Geometry: final body of the model. Coordinates: model frame, mm. A direction names the side the tool comes from. Coordinates: 2 decimals unless noted, no trailing zeros. Write each loop counter-clockwise with the first axis right and the second up, starting at its lowest first coordinate (ties: lowest second). Pieces come first, ordered by that corner, then holes.
from build123d import *

# Parameters (mm, degrees)
CHAMFER_1_SIZE = 1


with BuildPart() as part:
    # 草图1 → 旋转1 (revolve)
    with BuildSketch(Plane.XY):
        Polygon((0, 0), (6.325, 0), (6.325, 5), (8.5, 5), (8.5, 10), (3.66, 10), (3.66, 25), (0, 25), align=None)
    revolve(axis=Axis((0, 25, 0), (0, 1, 0)))

    # 倒角1
    chamfer_1_edges = [part.edges().sort_by_distance(p)[0] for p in [
        (-3.66, 25, 0),
    ]]
    chamfer(chamfer_1_edges, length=CHAMFER_1_SIZE)


solid = part.part
Item 1: Section C-C, the plane y = 15.5. Output: boundary loops of the cut face in (x, z).
Derived:
outline: circle Ø7.32 at (0, 0)
Item 2: Set-up query: faces 1 (the flat face through (6, 5, 3)), 2 (the flat face through (0, 0, 0)), 3 (the flat face through (4, 10, 0)). Return all of +Z, -Z, +X, -X, +Y, -Y with unobstructed straight access to the full face (end or side cutting, diameter ignored); none if empty.
Derived:
face 1: -Y
face 2: +Z, -Z, +X, -X, -Y
face 3: +Y
Item 3: Section B-B, the plane z = 0. Output: boundary loops of the cut face in (x, y) (3 decimals), plus the area to 3 significant figures.
Derived:
outline: (-8.5, 5) - (-6.325, 5) - (-6.325, 0) - (6.325, 0) - (6.325, 5) - (8.5, 5) - (8.5, 10) - (3.66, 10) - (3.66, 24) - (2.66, 25) - (-2.66, 25) - (-3.66, 24) - (-3.66, 10) - (-8.5, 10) - close
area: 257 mm2
Item 4: Section D-D, the plane x = -6. Output: boundary loops of the cut face in (y, z).
Derived:
outline: (0, -2) - (5, -2) - (5, -6.02) - (10, -6.02) - (10, 6.02) - (5, 6.02) - (5, 2) - (0, 2) - close
Item 5: Pin query (flat end, axial travel): pin 1 (5 mm diameter, centred on x = -1.5, y = 14.5, fed in from +Z); pin 2 (6 mm diameter, centred on y = 20, z = 0, fed in from +X); pin 3 (3 mm diameter, centred on x = -4.5, y = 19.5, fed in from +Z). Return the tip coordinate at first contact, or that it passes through.
Derived:
pin 1: stops at z = 3.66
pin 2: stops at x = 3.66
pin 3: stops at z = 2.1
Item 6: Material intervals for probe 1 along Y at (x, z) = (1.25, -4); probe 2 along Y at (x, z) = (-4.75, 5); probe 3 along Z at (x, y) = (-3.25, 5.5), sorted ascending.
Derived:
probe 1: y = 0 to 10
probe 2: y = 5 to 10
probe 3: z = -7.85 to 7.85
Item 7: Section A-A, the plane x = 0. Output: boundary loops of the cut face in (y, z) (3 decimals).
Derived:
outline: (0, -6.325) - (5, -6.325) - (5, -8.5) - (10, -8.5) - (10, -3.66) - (24, -3.66) - (25, -2.66) - (25, 2.66) - (24, 3.66) - (10, 3.66) - (10, 8.5) - (5, 8.5) - (5, 6.325) - (0, 6.325) - close
